Input: dimensioned drawing with shaded views. Units: mm. Origin: part minimum x, y, z. A direction names the side the tool comes from. Round coordinates to 2 decimals unless told otherwise and drop trailing zeros. Loops run counter-clockwise (first coordinate to the right, second up) from the corner with the lowest first, then second, coordinate; pieces in that order, holes last. Notation, with made-up numbers: M -35.5,39 L -24.5,39 A11 cw -24.5,59 Z; hole C 12,57.25 d6. An arc over 180 degrees is marked long. Put each result on its own line as item: value. Start each with the question number.
1) Section B-B on y = 85. Output: boundary loops of the cut face in (x, z), plus the area to 3 significant figures.
2) Reachability of the marked faces 1, 2 and 3 from +Z, -Z, +X, -X, +Y, -Y: full face, straight path, thin tool, end or side. Return the list, or none.
3) Line query: probe 1 along Z at (x, y) = (5, 92.5); probe 2 along Y at (x, z) = (28.5, 129). Output: solid intervals per line, ascending.
4) Pin query (flat end, axial travel): pin 1 (2 mm diameter, centred on x = 41.5, y = 69, fed in from +Z); pin 2 (3 mm diameter, centred on x = 21, z = 73.5, fed in from +Y); pin 3 (1.5 mm diameter, centred on y = 89.5, z = 48, fed in from -X). Return the tip coordinate at first contact, or that it passes through.
5) Section D-D on x = 30. Output: boundary loops of the cut face in (y, z), plus the area to 3 significant figures.
6) Section A-A on x = 19. Output: boundary loops of the cut face in (y, z).
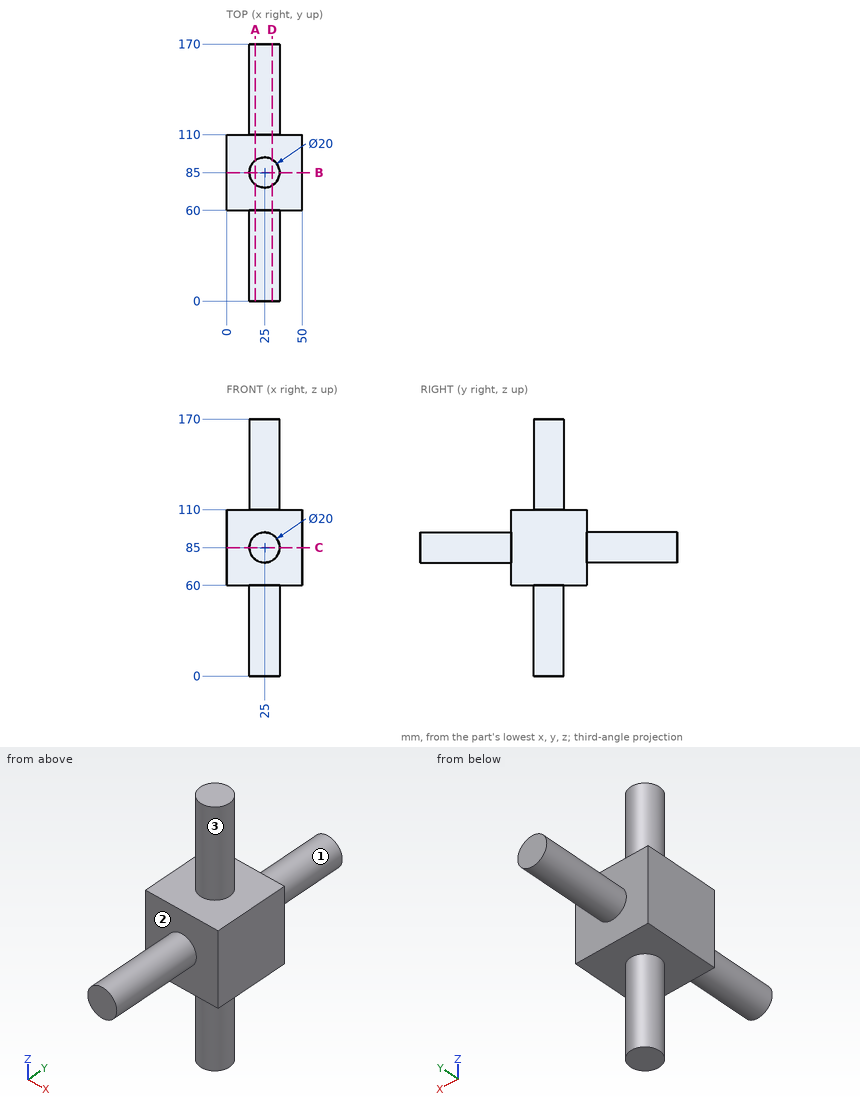
Geometry results:
1. outline: M 0,60 L 15,60 L 15,0 L 35,0 L 35,60 L 50,60 L 50,110 L 35,110 L 35,170 L 15,170 L 15,110 L 0,110 Z
1. area: 4,900 mm²
2. face 1: +Y
2. face 2: -Y
2. face 3: +Z
3. probe 1: z = 60 to 110
3. probe 2: y = 75.63 to 94.37
4. pin 1: stops at z = 110
4. pin 2: stops at y = 110
4. pin 3: stops at x = 15.73
5. outline: M 0,76.34 L 60,76.34 L 60,60 L 76.34,60 L 76.34,0 L 93.66,0 L 93.66,60 L 110,60 L 110,76.34 L 170,76.34 L 170,93.66 L 110,93.66 L 110,110 L 93.66,110 L 93.66,170 L 76.34,170 L 76.34,110 L 60,110 L 60,93.66 L 0,93.66 Z
5. area: 6,660 mm²
6. outline: M 0,77 L 60,77 L 60,60 L 77,60 L 77,0 L 93,0 L 93,60 L 110,60 L 110,77 L 170,77 L 170,93 L 110,93 L 110,110 L 93,110 L 93,170 L 77,170 L 77,110 L 60,110 L 60,93 L 0,93 Z
